from build123d import *

# Parameters (mm, degrees)
SKETCH_1_W          = 100
SKETCH_1_H          = 100
EXTRUDE_1_DEPTH     = 10
SKETCH_2_R          = 2.5
CUT_EXTRUDE_1_DEPTH = 10
SKETCH_3_R          = 2.5
CUT_EXTRUDE_2_DEPTH = 10
SKETCH_4_R          = 5
CUT_EXTRUDE_3_DEPTH = 11


with BuildPart() as part:
    # Эскиз1 → Бобышка-Вытянуть1 (new body)
    with BuildSketch(Plane(origin=(0, 0, 0), x_dir=(1, 0, 0), z_dir=(0, 1, 0))):
        Rectangle(SKETCH_1_W, SKETCH_1_H)
    extrude(amount=EXTRUDE_1_DEPTH)

    # Эскиз2 → Вырез-Вытянуть1 (cut)
    with BuildSketch(Plane.XY.offset(50)):
        with Locations((-25, 5)):
            Circle(SKETCH_2_R)
        with Locations((25, 5)):
            Circle(SKETCH_2_R)
    extrude(amount=-CUT_EXTRUDE_1_DEPTH, mode=Mode.SUBTRACT)

    # Эскиз3 → Вырез-Вытянуть2 (cut)
    with BuildSketch(Plane(origin=(0, 0, -50), x_dir=(-1, 0, 0), z_dir=(0, 0, -1))):
        with Locations((-25, 5)):
            Circle(SKETCH_3_R)
        with Locations((25, 5)):
            Circle(SKETCH_3_R)
    extrude(amount=-CUT_EXTRUDE_2_DEPTH, mode=Mode.SUBTRACT)

    # Эскиз4 → Вырез-Вытянуть3 (cut, through all)
    with BuildSketch(Plane(origin=(0, 10, 0), x_dir=(1, 0, 0), z_dir=(0, 1, 0))):
        Circle(SKETCH_4_R)
    extrude(amount=-CUT_EXTRUDE_3_DEPTH, mode=Mode.SUBTRACT)


solid = part.part
Verification items for the finished model (mm, model axes). A direction names the side the tool comes from. Round coordinates to 2 decimals unless told otherwise and drop trailing zeros. Loops run counter-clockwise (first coordinate to the right, second up) from the corner with the lowest first, then second, coordinate; pieces in that order, holes last. Notation, with made-up numbers: (14, 44.25) - (44, 44.25) arc R26 cw to (44, 73.25) - close; hole circle Ø4 at (10.25, 78.25). An arc over 180 degrees is marked (long way). Use one line per item in the form item = value.
1. Section check B-B on x = 0. Record the cut outline in (y, z).
A:
outline = (0, -50) - (10, -50) - (10, -5) - (0, -5) - close; (0, 5) - (10, 5) - (10, 50) - (0, 50) - close
2. Section check D-D on x = 25. Record the cut outline in (y, z).
A:
outline = (0, -50) - (2.5, -50) - (2.5, -40) - (7.5, -40) - (7.5, -50) - (10, -50) - (10, 50) - (7.5, 50) - (7.5, 40) - (2.5, 40) - (2.5, 50) - (0, 50) - close
3. Access from +Z, -Z, +X, -X, +Y, -Y to the whole of each face (thin tool, end or side, straight path). Record for faces 4 (the flat face through (50, 5, 1)), 5 (the cylindrical face through (23.16, 6.69, 45.07)), 6 (the flat face through (25, 5, -40)).
A:
face_4 = +Z, -Z, +X, +Y, -Y
face_5 = +Z
face_6 = -Z
4. Scan lines: probe 1 along X at (y, z) = (3.25, 0); probe 2 along Y at (x, z) = (-25, -45.75). Record each from-to range of solid material in increasing order.
A:
probe_1 = -50 to -5, 5 to 50
probe_2 = 0 to 2.5, 7.5 to 10
5. Draft check along Y on faces 1 (the cylindrical face through (26.84, 6.69, -45.07)), 2 (the cylindrical face through (-1.08, 5.07, 4.88)), 3 (the flat face through (-1, 10, -12)). Enter one of: pulls with the +Y half, pulls with the -Y half, needs draft (parallel to the pull), parting line crosses it, or undercut.
A:
face_1 = undercut
face_2 = needs draft
face_3 = pulls with the +Y half
6. Section check C-C on y = 5. Record the cut outline in (x, z).
A:
outline = (-50, -50) - (-27.5, -50) - (-27.5, -40) - (-22.5, -40) - (-22.5, -50) - (22.5, -50) - (22.5, -40) - (27.5, -40) - (27.5, -50) - (50, -50) - (50, 50) - (27.5, 50) - (27.5, 40) - (22.5, 40) - (22.5, 50) - (-22.5, 50) - (-22.5, 40) - (-27.5, 40) - (-27.5, 50) - (-50, 50) - close; hole circle Ø10 at (0, 0)
7. Gauge pin test, flat ends, axial feed: pin 1 Ø1.5 at (x, y) = (26, 5.5) entering from -Z; pin 2 Ø1.5 at (x, y) = (24, 5.5) entering from +Z. Record the tip position at first contact, or that the pin passes through.
A:
pin_1 = -40
pin_2 = 40
8. Section check A-A on z = 3. Record the cut outline in (x, y).
A:
outline = (-50, 0) - (-4, 0) - (-4, 10) - (-50, 10) - close; (4, 0) - (50, 0) - (50, 10) - (4, 10) - close
